from build123d import *

# Parameters (mm, degrees)
F0_R      = 41.5
F1_DEPTH  = 2
F3_DEPTH  = 21
F4_R      = 41.5
F5_DEPTH  = 2
F6_R      = 4
F6_R_2    = 2.5
F7_DEPTH  = 2
F8_DEPTH  = 7
F10_R     = 41.5
F11_DEPTH = 2
F13_R     = 0.5
F14_DEPTH = 2
F15_DEPTH = 6


with BuildPart() as f1:
    # F0 (on Right) → F1 (new body)
    with BuildSketch(Plane.YZ):
        Circle(F0_R)
    extrude(amount=F1_DEPTH)

    # F2 (on face) → F3 (join)
    with BuildSketch(Plane.YZ.offset(2)):
        with BuildLine():
            ThreePointArc((9.8646073485, -2.5262456751), (10.1030481106, -1.2731120236), (10.1829463001, 0))
            ThreePointArc((10.1829463001, 0), (10.037899881, 1.7125890722), (9.6068927211, 3.376389728))
            ThreePointArc((9.6068927211, 3.376389728), (9.2288835267, 4.3034990647), (8.7616561977, 5.189005302))
            ThreePointArc((8.7616561977, 5.189005302), (6.8289840342, 7.5536330604), (4.2820740528, 9.2388439297))
            ThreePointArc((4.2820740528, 9.2388439297), (3.3540046296, 9.6147307968), (2.3935052702, 9.8976526446))
            ThreePointArc((2.3935052702, 9.8976526446), (-0.5124946806, 10.1700415217), (-3.376389728, 9.6068927211))
            ThreePointArc((-3.376389728, 9.6068927211), (-4.3034990647, 9.2288835267), (-5.189005302, 8.7616561977))
            ThreePointArc((-5.189005302, 8.7616561977), (-7.507655529, 6.879498805), (-9.1805670618, 4.4056309167))
            ThreePointArc((-9.1805670618, 4.4056309167), (-9.5688394961, 3.482772753), (-9.8646073485, 2.5262456751))
            ThreePointArc((-9.8646073485, 2.5262456751), (-10.1732543916, -0.4441738792), (-9.6068927211, -3.376389728))
            ThreePointArc((-9.6068927211, -3.376389728), (-9.2288835267, -4.3034990647), (-8.7616561977, -5.189005302))
            ThreePointArc((-8.7616561977, -5.189005302), (-6.879498805, -7.507655529), (-4.4056309167, -9.1805670618))
            ThreePointArc((-4.4056309167, -9.1805670618), (-3.482772753, -9.5688394961), (-2.5262456751, -9.8646073485))
            ThreePointArc((-2.5262456751, -9.8646073485), (0.4441738792, -10.1732543916), (3.376389728, -9.6068927211))
            ThreePointArc((3.376389728, -9.6068927211), (4.3034990647, -9.2288835267), (5.189005302, -8.7616561977))
            ThreePointArc((5.189005302, -8.7616561977), (7.507655529, -6.879498805), (9.1805670618, -4.4056309167))
            ThreePointArc((9.1805670618, -4.4056309167), (9.5688394961, -3.482772753), (9.8646073485, -2.5262456751))
        make_face()
        with BuildLine():
            ThreePointArc((2.3935052702, 9.8976526446), (3.3540046296, 9.6147307968), (4.2820740528, 9.2388439297))
            Line((4.2820740528, 9.2388439297), (15.0026191162, 38.6932994155))
            ThreePointArc((15.0026191162, 38.6932994155), (14.0658892352, 39.043575144), (13.1209909217, 39.3711772396))
            Line((13.1209909217, 39.3711772396), (2.3935052702, 9.8976526446))
        make_face()
        with BuildLine():
            ThreePointArc((-5.189005302, 8.7616561977), (-4.3034990647, 9.2288835267), (-3.376389728, 9.6068927211))
            Line((-3.376389728, 9.6068927211), (-16.6272575496, 38.0234704673))
            ThreePointArc((-16.6272575496, 38.0234704673), (-17.5386578622, 37.611773162), (-18.4398731237, 37.1782339438))
            Line((-18.4398731237, 37.1782339438), (-5.189005302, 8.7616561977))
        make_face()
        with BuildLine():
            ThreePointArc((8.7616561977, 5.189005302), (9.2288835267, 4.3034990647), (9.6068927211, 3.376389728))
            Line((9.6068927211, 3.376389728), (38.0234704673, 16.6272575496))
            ThreePointArc((38.0234704673, 16.6272575496), (37.611773162, 17.5386578622), (37.1782339438, 18.4398731237))
            Line((37.1782339438, 18.4398731237), (8.7616561977, 5.189005302))
        make_face()
        with BuildLine():
            Line((39.3279406642, -13.2500220043), (9.8646073485, -2.5262456751))
            ThreePointArc((9.8646073485, -2.5262456751), (9.5688394961, -3.482772753), (9.1805670618, -4.4056309167))
            Line((9.1805670618, -4.4056309167), (38.6439003775, -15.1294072458))
            ThreePointArc((38.6439003775, -15.1294072458), (38.9972437626, -14.193835948), (39.3279406642, -13.2500220043))
        make_face()
        with BuildLine():
            Line((18.4398731237, -37.1782339438), (5.189005302, -8.7616561977))
            ThreePointArc((5.189005302, -8.7616561977), (4.3034990647, -9.2288835267), (3.376389728, -9.6068927211))
            Line((3.376389728, -9.6068927211), (16.6272575496, -38.0234704673))
            ThreePointArc((16.6272575496, -38.0234704673), (17.5386578622, -37.611773162), (18.4398731237, -37.1782339438))
        make_face()
        with BuildLine():
            Line((-13.2500220043, -39.3279406642), (-2.5262456751, -9.8646073485))
            ThreePointArc((-2.5262456751, -9.8646073485), (-3.482772753, -9.5688394961), (-4.4056309167, -9.1805670618))
            Line((-4.4056309167, -9.1805670618), (-15.1294072458, -38.6439003775))
            ThreePointArc((-15.1294072458, -38.6439003775), (-14.193835948, -38.9972437626), (-13.2500220043, -39.3279406642))
        make_face()
        with BuildLine():
            ThreePointArc((-9.8646073485, 2.5262456751), (-9.5688394961, 3.482772753), (-9.1805670618, 4.4056309167))
            Line((-9.1805670618, 4.4056309167), (-38.6439003775, 15.1294072458))
            ThreePointArc((-38.6439003775, 15.1294072458), (-38.9972437626, 14.193835948), (-39.3279406642, 13.2500220043))
            Line((-39.3279406642, 13.2500220043), (-9.8646073485, 2.5262456751))
        make_face()
        with BuildLine():
            Line((-37.1782339438, -18.4398731237), (-8.7616561977, -5.189005302))
            ThreePointArc((-8.7616561977, -5.189005302), (-9.2288835267, -4.3034990647), (-9.6068927211, -3.376389728))
            Line((-9.6068927211, -3.376389728), (-38.0234704673, -16.6272575496))
            ThreePointArc((-38.0234704673, -16.6272575496), (-37.611773162, -17.5386578622), (-37.1782339438, -18.4398731237))
        make_face()
    extrude(amount=F3_DEPTH)

    # F4 (on face) → F5 (join)
    with BuildSketch(Plane.YZ.offset(23)):
        Circle(F4_R)
    extrude(amount=F5_DEPTH)

    # F6 (on face) → F7 (join)
    with BuildSketch(Plane(origin=(0, 0, 0), x_dir=(0, -1, 0), z_dir=(-1, 0, 0))):
        Circle(F6_R)
        Circle(F6_R_2, mode=Mode.SUBTRACT)
    extrude(amount=F7_DEPTH)

    # F8 (add): a face of the model
    f8_faces = [f1.faces().sort_by_distance(p)[0] for p in [
        (0, 0, 0),
    ]]
    extrude(f8_faces, amount=F8_DEPTH)

    # F10 (on face) → F11 (join)
    with BuildSketch(Plane.YZ.offset(25)):
        Circle(F10_R)
    extrude(amount=F11_DEPTH)

    # F13 (on face) → F14 (cut)
    with BuildSketch(Plane.YZ.offset(27)):
        with BuildLine():
            Line((0, -2.5), (8.1875, -1.4882351125))
            ThreePointArc((8.1875, -1.4882351125), (9.5, 0), (8.1875, 1.4882351125))
            Line((8.1875, 1.4882351125), (0, 2.5197631534))
            Line((0, 2.5197631534), (-8.1875, 1.4882351125))
            ThreePointArc((-8.1875, 1.4882351125), (-9.5, 0), (-8.1875, -1.4882351125))
            Line((-8.1875, -1.4882351125), (0, -2.5))
        make_face()
        with Locations((-6, 0)):
            Circle(F13_R, mode=Mode.SUBTRACT)
        with Locations((-3, 0)):
            Circle(F13_R, mode=Mode.SUBTRACT)
        with Locations((3, 0)):
            Circle(F13_R, mode=Mode.SUBTRACT)
        with Locations((6, 0)):
            Circle(F13_R, mode=Mode.SUBTRACT)
    extrude(amount=-F14_DEPTH, mode=Mode.SUBTRACT)

    # F15 (cut): faces of the model
    f15_faces = [f1.faces().sort_by_distance(p)[0] for p in [
        (27, -3, 0),
        (27, -6, 0),
        (27, 3, 0),
        (27, 6, 0),
    ]]
    extrude(f15_faces, amount=-F15_DEPTH, mode=Mode.SUBTRACT)


solid = f1.part
Model file for the job. Use its own axes, mm. A direction names the side the tool comes from. Round coordinates to 2 decimals unless told otherwise and drop trailing zeros. Loops run counter-clockwise (first coordinate to the right, second up) from the corner with the lowest first, then second, coordinate; pieces in that order, holes last.
1. Mould opens along X. For faces 5 (the cylindrical face through (26, 9.5, 0)), 6 (the flat face through (25, 0, 0)), 7 (the flat face through (2, 29, 2)) say: +X half, -X half, draft (parallel to the pull), parting line (faces both ways), or undercut.
Check values:
face 5: draft
face 6: +X half
face 7: undercut
2. Wall check: probe 1 along X at (y, z) = (-25, -18); probe 2 along Z at (x, y) = (10, -18); probe 3 along X at (y, z) = (-2.5, -4). Give the ranges that are in metal, low to high.
Check values:
probe 1: x = 0 to 2, 23 to 27
probe 2: z = -9.5 to -7.29, 5.49 to 7.62, 36.23 to 37.39
probe 3: x = 0 to 27
3. Band-saw the part on D-D, the plane x = -3. List the corners of the cut face in (y, z), and give its area (3 significant figures).
Check values:
outline: circle Ø5 at (0, 0)
area: 19.6 mm2
4. Tool access for faces 1 (the flat face through (2, -2, 29)), 2 (the cylindrical face through (12.353, 0.402, -10.175)), 3 (the flat face through (12.353, 11.907, -23.169)), 4 (the cylindrical face through (26, -9.5, 0)): list every direction of +Z, -Z, +X, -X, +Y, -Y with a clear straight run to the whole face (end or side of a thin tool).
Check values:
face 1: +Z
face 2: -Z
face 3: none
face 4: +X
5. Drop flat-ended pins along their axis: P1, Ø24, axis at y = 4, z = 30.5, coming from the -X side; P2, Ø0.5, axis at y = 3, z = 0, coming from the +X side; P3, Ø4, axis at x = 19.5, z = 9.5, coming from the +Y side; P4, Ø5.5, axis at y = -1, z = -0.5, coming from the +X side. Give the stop position or say it passes through.
Check values:
P1: stops at x = 0
P2: stops at x = 21
P3: stops at y = 27.03
P4: stops at x = 27
6. Band-saw the part on B-B, the plane y = 33. List the corners of the cut face in (x, z).
Check values:
outline: (0, -25.16) - (2, -25.16) - (2, -13.08) - (23, -13.08) - (23, -25.16) - (27, -25.16) - (27, 25.16) - (23, 25.16) - (23, 16.49) - (2, 16.49) - (2, 25.16) - (0, 25.16) - close; hole (2, -10.95) - (23, -10.95) - (23, 14.28) - (2, 14.28) - close
7. Band-saw the part on C-C, the plane z = 28. List the corners of the cut face in (x, y).
Check values:
outline: (0, -30.63) - (2, -30.63) - (2, -14.16) - (23, -14.16) - (23, -30.63) - (27, -30.63) - (27, 30.63) - (23, 30.63) - (23, 11.11) - (2, 11.11) - (2, 30.63) - (0, 30.63) - close; hole (2, -11.95) - (23, -11.95) - (23, 8.98) - (2, 8.98) - close
